from build123d import *

# Parameters (mm, degrees)
F1_DEPTH = 484
F3_W     = 130
F3_H     = 80
F3_R     = 6
F4_DEPTH = 8
F6_W     = 130
F6_H     = 80
F6_R     = 6
F7_DEPTH = 8


with BuildPart() as f1:
    # F0 (on Front) → F1 (new body)
    with BuildSketch(Plane.XZ):
        with BuildLine():
            ThreePointArc((40, 34), (38.2426406871, 38.2426406871), (34, 40))
            Line((34, 40), (-34, 40))
            ThreePointArc((-34, 40), (-38.2426406871, 38.2426406871), (-40, 34))
            Line((-40, 34), (-40, -34))
            ThreePointArc((-40, -34), (-38.2426406871, -38.2426406871), (-34, -40))
            Line((-34, -40), (34, -40))
            ThreePointArc((34, -40), (38.2426406871, -38.2426406871), (40, -34))
            Line((40, -34), (40, 34))
        make_face()
        with BuildLine():
            ThreePointArc((-36, 34), (-35.4142135624, 35.4142135624), (-34, 36))
            Line((-34, 36), (34, 36))
            ThreePointArc((34, 36), (35.4142135624, 35.4142135624), (36, 34))
            Line((36, 34), (36, -34))
            ThreePointArc((36, -34), (35.4142135624, -35.4142135624), (34, -36))
            Line((34, -36), (-34, -36))
            ThreePointArc((-34, -36), (-35.4142135624, -35.4142135624), (-36, -34))
            Line((-36, -34), (-36, 34))
        make_face(mode=Mode.SUBTRACT)
    extrude(amount=-F1_DEPTH)

    # F3 (on offset) → F4 (join)
    with BuildSketch(Plane.XZ.offset(8)):
        Rectangle(F3_W, F3_H)
        with Locations((-53, -28)):
            Circle(F3_R, mode=Mode.SUBTRACT)
        with Locations((53, -28)):
            Circle(F3_R, mode=Mode.SUBTRACT)
        with Locations((-53, 28)):
            Circle(F3_R, mode=Mode.SUBTRACT)
        with Locations((53, 28)):
            Circle(F3_R, mode=Mode.SUBTRACT)
    extrude(amount=-F4_DEPTH)

    # F6 (on offset) → F7 (join)
    with BuildSketch(Plane(origin=(0, 492, 0), x_dir=(-1, 0, 0), z_dir=(0, 1, 0))):
        Rectangle(F6_W, F6_H)
        with Locations((-53, -28)):
            Circle(F6_R, mode=Mode.SUBTRACT)
        with Locations((53, -28)):
            Circle(F6_R, mode=Mode.SUBTRACT)
        with Locations((-53, 28)):
            Circle(F6_R, mode=Mode.SUBTRACT)
        with Locations((53, 28)):
            Circle(F6_R, mode=Mode.SUBTRACT)
    extrude(amount=-F7_DEPTH)


solid = f1.part
Can you work these out from the model? Positions are in its coordinate system, mm. A direction names the side the tool comes from. Coordinates: 2 decimals unless noted, no trailing zeros. Write each loop counter-clockwise with the first axis right and the second up, starting at its lowest first coordinate (ties: lowest second). Pieces come first, ordered by that corner, then holes. Notation, with made-up numbers: (11, 54) - (52, 54) arc R24 cw to (52, 74) - close; hole circle Ø8 at (-5.5, 43.5). An arc over 180 degrees is marked (long way). Return JSON: item names as keys, results as strings. Group by question number.
Item 1: We'd pull the mould along Z, two halves only. Please class faces 1 (the face through (-57.76, -4.06, -31.65)), 2 (the face through (-53, 484, 1)), 3 (the face through (1, 246, -40)): pulls with the +Z half, pulls with the -Z half, needs draft (parallel to the pull), parting line crosses it, or undercut.
Item 2: Please list where these lines run through material, in increasing order: probe 1 along Z at (x, y) = (-53, 489.5); probe 2 along Z at (x, y) = (-6, 408); probe 3 along Y at (x, z) = (-17, -17.5).
Item 3: If we section it at D-D (y = 36.5): Write out the boundary of the cut face in (x, z).
Item 4: If we section it at C-C (x = 53): Write out the boundary of the cut face in (y, z).
Item 5: I'm going to push flat-ended pins straight in: pin 1 Ø12 at (y, z) = (426, -13.5) entering from +X; pin 2 Ø7 at (x, z) = (53, 28) entering from +Y. Where does each tip first touch, or does it pass through?
Item 6: Which directions (+Z, -Z, +X, -X, +Y, -Y) give clear straight access to the entire face, cutting with the end or side of a thin tool? Please do faces 4 (the face through (65, 488, -1)), 5 (the face through (40, 239, 0)), 6 (the face through (0, 239, 36)).
Item 7: If we section it at A-A (z = -28): Count the separate pieces of the cut face and the enclosed holes in it, then the cut area to 3 significant figures.
Item 8: If we section it at B-B (z = -2): Write out the boundary of the cut face in (x, y), then the cut area to 3 significant figures.
Return value:
{
 "1": {"face 1": "undercut", "face 2": "needs draft", "face 3": "pulls with the -Z half"},
 "2": {"probe 1": "z = -40 to -34, -22 to 22, 34 to 40", "probe 2": "z = -40 to -36, 36 to 40", "probe 3": "y = -8 to 0, 484 to 492"},
 "3": {"outline": "(-40, -34) arc R6 ccw to (-34, -40) - (34, -40) arc R6 ccw to (40, -34) - (40, 34) arc R6 ccw to (34, 40) - (-34, 40) arc R6 ccw to (-40, 34) - close; hole (-36, -34) arc R2 ccw to (-34, -36) - (34, -36) arc R2 ccw to (36, -34) - (36, 34) arc R2 ccw to (34, 36) - (-34, 36) arc R2 ccw to (-36, 34) - close"},
 "4": {"outline": "(-8, -40) - (0, -40) - (0, -34) - (-8, -34) - close; (-8, -22) - (0, -22) - (0, 22) - (-8, 22) - close; (-8, 34) - (0, 34) - (0, 40) - (-8, 40) - close; (484, -40) - (492, -40) - (492, -34) - (484, -34) - close; (484, -22) - (492, -22) - (492, 22) - (484, 22) - close; (484, 34) - (492, 34) - (492, 40) - (484, 40) - close"},
 "5": {"pin 1": "stops at x = 40", "pin 2": "passes through"},
 "6": {"face 4": "+Z, -Z, +X, +Y, -Y", "face 5": "+Z, -Z, +X", "face 6": "none"},
 "7": {"separate pieces": "5", "enclosed holes": "1", "area": "5,570 mm^2"},
 "8": {"outline": "(-65, -8) - (65, -8) - (65, 0) - (40, 0) - (40, 484) - (65, 484) - (65, 492) - (-65, 492) - (-65, 484) - (-40, 484) - (-40, 0) - (-65, 0) - close; hole (-36, 0) - (36, 0) - (36, 484) - (-36, 484) - close", "area": "5,950 mm^2"}
}
